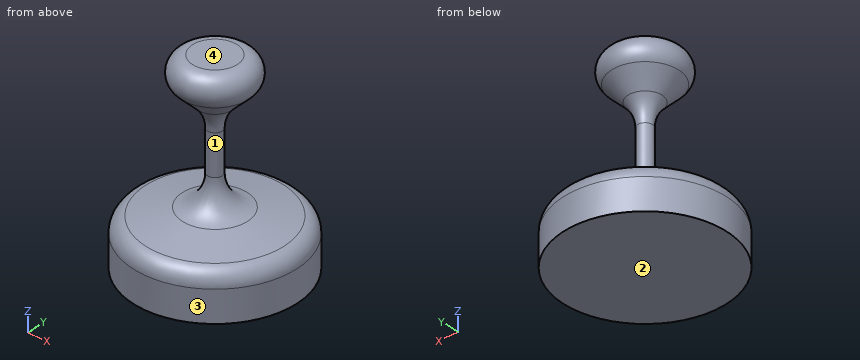
```python
from build123d import *


with BuildPart() as f1:
    # F0 (on Right) → F1 (revolve)
    with BuildSketch(Plane.YZ):
        with BuildLine():
            Line((-51.330089, -73.760578), (0, -73.760578))
            Line((0, -73.760578), (0, 47.362838))
            Line((0, 47.362838), (-14.093457, 47.362838))
            ThreePointArc((-14.093457, 47.362838), (-23.352265, 41.140996), (-21.089705, 30.217734))
            Line((-21.089705, 30.217734), (-10.693563, 20.038178))
            ThreePointArc((-10.693563, 20.038178), (-6.249005, 13.498779), (-4.686059, 5.74797))
            Line((-4.686059, 5.74797), (-4.686059, -19.709873))
            ThreePointArc((-4.686059, -19.709873), (-9.122987, -32.271354), (-20.46514, -39.259396))
            Line((-20.46514, -39.259396), (-43.440548, -44.219994))
            ThreePointArc((-43.440548, -44.219994), (-49.111624, -47.714015), (-51.330089, -53.994756))
            Line((-51.330089, -53.994756), (-51.330089, -73.760578))
        make_face()
    revolve(axis=Axis((0, 0, -13.19887), (0, 0, -1)))


solid = f1.part
```
Part model, mm, in its own coordinate system. Face numbers are marked on the shaded views. Coordinates: 2 decimals unless noted, no trailing zeros. Order: outer loops, then holes, each group sorted by start corner. A loop starts at its lowest first (then second) coordinate and runs counter-clockwise, first axis right, second up. Notation, with made-up numbers: (-27.75, -37) - (15.25, -37) arc R15 cw to (15.25, -13) - close; hole circle Ø5 at (5.5, 8). An arc over 180 degrees is marked (long way). Return JSON: item names as keys, results as strings. Group by question number.
Item 1: Cut at C-C (z = 26). List the corners of the cut face in (x, y).
Item 2: Drill centre lines: probe 1 along Z at (x, y) = (-7, -15); probe 2 along Z at (x, y) = (-9.5, -1); probe 3 along Z at (x, y) = (-20.5, 37). Where is each one in solid material? Low to high. Write a range as from..to.
Item 3: Pin check, flat tips, straight feed: pin 1 (8 mm diameter, centred on x = -8.5, z = -46, fed in from -Y); pin 2 (8 mm diameter, centred on y = 2, z = 20.5, fed in from +X). Stop position of each tip, or through.
Item 4: Pull direction Z, two halves, no side cores. Call the marked faces 1, 2, 3 and 4: pulls with the +Z half, pulls with the -Z half, needs draft (parallel to the pull), parting line crosses it, or undercut.
Item 5: Cut at A-A (y = 0). List the corners of the cut face in (x, z).
Item 6: Cut at D-D (z = -51). List the corners of the cut face in (x, y), plus the area to 3 significant figures.
Check values:
{
 "1": {"outline": "circle Ø33.56 at (0, 0)"},
 "2": {"probe 1": "z = -73.76..-37.98, 25.78..47.06", "probe 2": "z = -73.76..-32.79, 18.82..47.36", "probe 3": "z = -73.76..-43.97"},
 "3": {"pin 1": "stops at y = -49.88", "pin 2": "stops at x = 15.15"},
 "4": {"face 1": "undercut", "face 2": "pulls with the -Z half", "face 3": "needs draft", "face 4": "pulls with the +Z half"},
 "5": {"outline": "(-51.33, -73.76) - (51.33, -73.76) - (51.33, -53.99) arc R10 ccw to (43.44, -44.22) - (20.47, -39.26) arc R20 cw to (4.69, -19.71) - (4.69, 5.75) arc R20 cw to (10.69, 20.04) - (21.09, 30.22) arc R10 ccw to (14.09, 47.36) - (-14.09, 47.36) arc R10 ccw to (-21.09, 30.22) - (-10.69, 20.04) arc R20 cw to (-4.69, 5.75) - (-4.69, -19.71) arc R20 cw to (-20.47, -39.26) - (-43.44, -44.22) arc R10 ccw to (-51.33, -53.99) - close"},
 "6": {"outline": "circle Ø101.74 at (0, 0)", "area": "8,130 mm2"}
}
